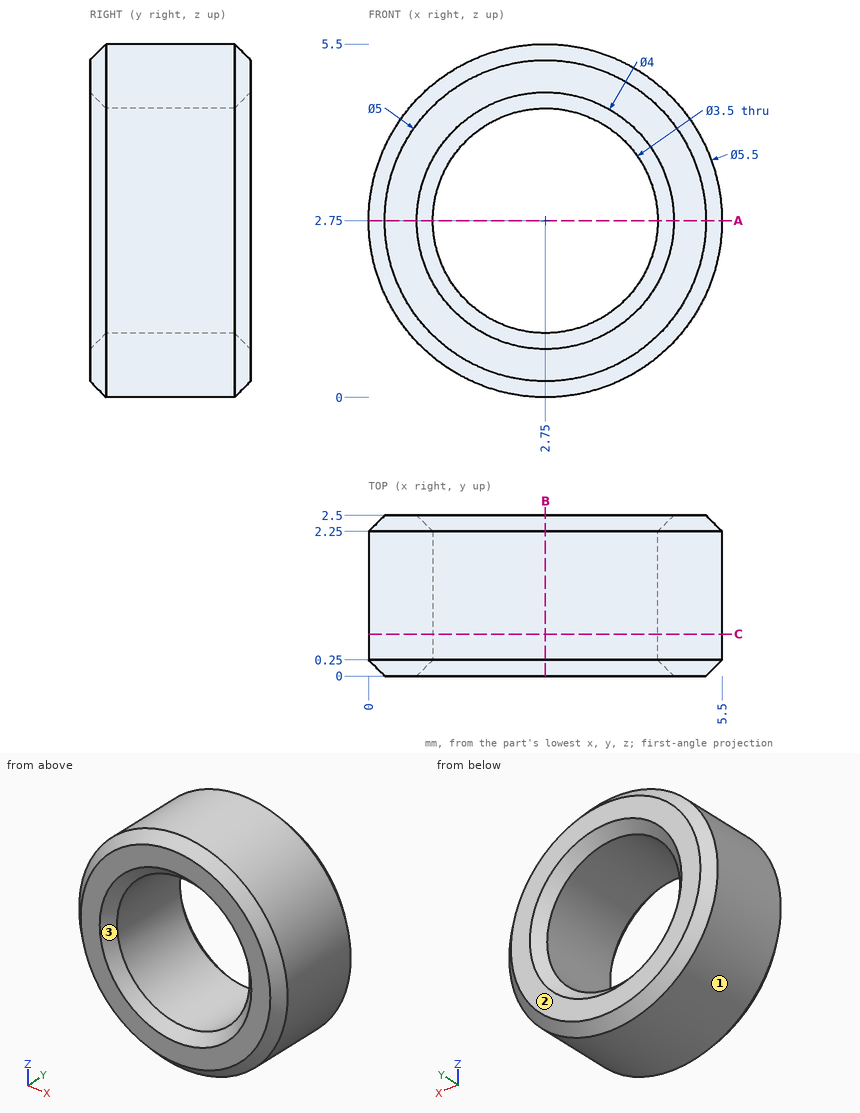
Answer from the drawing. Dimensions are ordinates in mm from the lowest x, y and z of the part. Coordinates: 2 decimals unless noted, no trailing zeros. Loops run counter-clockwise (first coordinate to the right, second up) from the corner with the lowest first, then second, coordinate; pieces in that order, holes last.
Q1. The part is cut by section A-A on z = 2.75. Write down the section's boundary in (x, y).
Q2. Consider probe 1 along X at (y, z) = (1.65, 2.75); probe 2 along X at (y, z) = (1.8, 3.6). Determine where each line is inside the solid, lowest interval first.
Q3. This flat-tipped pin is pushed along its axis until it touches: pin 1 Ø3 at (x, z) = (2.75, 2.75) entering from -Y. Where does it stop, or does it pass through?
Q4. The mould has two halves that part along X. Classify the marked faces 1, 2 and 3: +X half, -X half, draft (parallel to the pull), parting line (faces both ways), or undercut.
Q5. The part is cut by section B-B on x = 2.75. Write down the section's boundary in (y, z), and give its area (3 significant figures).
Q6. The part is cut by section C-C on y = 0.65. Write down the section's boundary in (x, z).
Results below:
1. outline: (0, 0.25) - (0.25, 0) - (0.75, 0) - (1, 0.25) - (1, 2.25) - (0.75, 2.5) - (0.25, 2.5) - (0, 2.25) - close; (4.5, 0.25) - (4.75, 0) - (5.25, 0) - (5.5, 0.25) - (5.5, 2.25) - (5.25, 2.5) - (4.75, 2.5) - (4.5, 2.25) - close
2. probe 1: x = 0 to 1, 4.5 to 5.5
2. probe 2: x = 0.13 to 1.22, 4.28 to 5.37
3. pin 1: passes through
4. face 1: parting line
4. face 2: draft
4. face 3: undercut
5. outline: (0, 0.25) - (0.25, 0) - (2.25, 0) - (2.5, 0.25) - (2.5, 0.75) - (2.25, 1) - (0.25, 1) - (0, 0.75) - close; (0, 4.75) - (0.25, 4.5) - (2.25, 4.5) - (2.5, 4.75) - (2.5, 5.25) - (2.25, 5.5) - (0.25, 5.5) - (0, 5.25) - close
5. area: 4.75 mm2
6. outline: circle Ø5.5 at (2.75, 2.75); hole circle Ø3.5 at (2.75, 2.75)
